Can you work these out from the model? Positions are in its coordinate system, mm. Face numbers are marked on the shaded views. A direction names the side the tool comes from. Coordinates: 2 decimals unless noted, no trailing zeros. Order: outer loops, then holes, each group sorted by start corner. A loop starts at its lowest first (then second) coordinate and runs counter-clockwise, first axis right, second up. Notation, with made-up numbers: (70.5, 40.25) -> (113.5, 40.25) arc R21 ccw to (113.5, 74.25) -> close; hole circle Ø4 at (58.5, 36.25). An arc over 180 degrees is marked (long way). Answer in a Markdown table with one row per item.
```python
from build123d import *

# Parameters (mm, degrees)
F0_W     = 10.3
F0_H     = 10.3
F0_W_2   = 0.75
F0_H_2   = 8
F1_DEPTH = 9


with BuildPart() as f1:
    # F0 (on Front) → F1 (new body)
    with BuildSketch(Plane.XZ):
        Polygon((-22.7488241771, 49.3360479977), (-30.7488241771, 49.3360479977), (-30.7488241771, 41.3360479977), (-30.7488241771, -60.2917829884), (-30.7488241771, -67.4802789781), (109.2511758229, -4.6212578508), align=None)
        with Locations((-20.7488241771, -45.5300207496)):
            Rectangle(F0_W, F0_H, mode=Mode.SUBTRACT)
        with Locations((-20.7488241771, 34.4699792504)):
            Rectangle(F0_W, F0_H, mode=Mode.SUBTRACT)
        Polygon((-8.6376664854, -26.1920627463), (-8.6376664854, 27.3630689768), (10.1197385162, 19.6956520177), (19.9698888285, 15.6692310097), (34.8834536025, 9.57305089), (43.9300421098, 5.8750998068), (64.9299837446, -2.708993175), (34.8072479351, -16.4188460197), (21.847787114, -22.3171250448), (0.4639824944, -32.0496014191), (-8.6376664854, -36.1920627463), align=None, mode=Mode.SUBTRACT)
        with Locations((81.7206834825, -5.5300207496)):
            Rectangle(F0_W, F0_H, mode=Mode.SUBTRACT)
        Polygon((19.9698888285, 15.6692310097), (10.1197385162, 19.6956520177), (-8.6376664854, -26.1920627463), (-8.6376664854, -36.1920627463), (0.4639824944, -32.0496014191), align=None)
        Polygon((-30.7488241771, 41.3360479977), (-30.7488241771, 49.3360479977), (-59.7488241771, 49.3360479977), (-59.7488241771, 29.3360479977), (-51.7488241771, 29.3360479977), (-51.7488241771, 37.3360479977), (-51.7488241771, 41.3360479977), align=None)
        Polygon((43.9300421098, 5.8750998068), (34.8834536025, 9.57305089), (21.847787114, -22.3171250448), (34.8072479351, -16.4188460197), (34.8834536025, -16.2562809986), (41.1210870837, -0.9966677438), align=None)
        with Locations((-51.3738241771, 33.3360479977)):
            Rectangle(F0_W_2, F0_H_2)
    extrude(amount=F1_DEPTH)


solid = f1.part
```
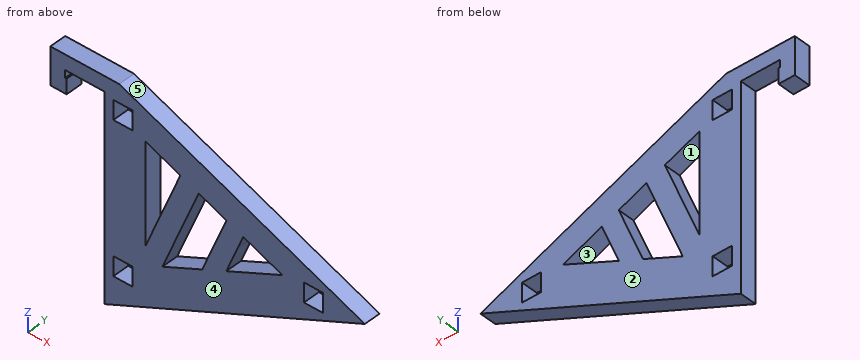
(1) I need wall thicknesses on line 1 (X direction, y = -5.5, z = 5); line 2 (X direction, y = -4.75, z = 10.5); line 3 (Z direction, x = 4, y = -6). Which ranges of each line are inside material? Lowest first, please. Write a range as [from, to].
Response values:
| item | result |
|---|---|
| line 1 | [-30.75, -8.64], [4.11, 15.61], [33.01, 43.57], [46.07, 85.71] |
| line 2 | [-30.75, -8.64], [6.36, 17.86], [32.62, 72.26] |
| line 3 | [-51.88, -30.44], [-23.4, 4.72], [22.2, 38.4] |
(2) Will these pins go through, and if not, where does the flat tip stop? pin 1 Ø2.5 at (x, y) = (-20, -4.5) entering from +Z; pin 2 Ø4.5 at (y, z) = (-6.5, -31) entering from -X; pin 3 Ø3 at (x, y) = (24.5, -4) entering from +Z.
Response values:
| item | result |
|---|---|
| pin 1 | z = 48.72 |
| pin 2 | x = -30.75 |
| pin 3 | z = 30.64 |
(3) We'd pull the mould along Z, two halves only. Please class the marked faces 3, 4 and 5: +Z half, -Z half, draft (parallel to the pull), parting line (faces both ways), or undercut.
Response values:
| item | result |
|---|---|
| face 3 | undercut |
| face 4 | draft |
| face 5 | +Z half |
(4) Suppose I cut it at A-A (y = -1.5). Count the separate pieces of the cut face and the enclosed holes in it, and give its area (3 significant figures).
Response values:
| item | result |
|---|---|
| separate pieces | 1 |
| enclosed holes | 6 |
| area | 6,940 mm2 |
(5) On a 3-axis mill with a long thin cutter (end or side, diameter ignored), from which of +Z, -Z, +X, -X, +Y, -Y can I reach the whole of each face in a straight line? I mean the marked faces 1 and 2. Say none if no direction works.
Response values:
| item | result |
|---|---|
| face 1 | +Y, -Y |
| face 2 | +Z, -Z, +X, -X, +Y |
(6) Suppose I cut it at B-B (x = 56). Please give me the cut outline in (y, z).
Response values:
| item | result |
|---|---|
| outline | (-9, -28.53) -> (0, -28.53) -> (0, -6.77) -> (-9, -6.77) -> close; (-9, 0.94) -> (0, 0.94) -> (0, 17.15) -> (-9, 17.15) -> close |
(7) Suppose I cut it at D-D (z = -6.5). Please give me the cut outline in (x, y).
Response values:
| item | result |
|---|---|
| outline | (-30.75, -9) -> (-8.64, -9) -> (-8.64, 0) -> (-30.75, 0) -> close; (-0.59, -9) -> (10.91, -9) -> (10.91, 0) -> (-0.59, 0) -> close; (28.31, -9) -> (38.87, -9) -> (38.87, 0) -> (28.31, 0) -> close; (56.6, -9) -> (76.57, -9) -> (76.57, 0) -> (56.6, 0) -> close; (86.87, -9) -> (105.07, -9) -> (105.07, 0) -> (86.87, 0) -> close |
(8) Suppose I cut it at C-C (z = -48). Please give me the cut outline in (x, y).
Response values:
| item | result |
|---|---|
| outline | (-30.75, -9) -> (-25.9, -9) -> (-25.9, 0) -> (-30.75, 0) -> close; (-15.6, -9) -> (12.64, -9) -> (12.64, 0) -> (-15.6, 0) -> close |
